from build123d import *

# Parameters (mm, degrees)
F0_W     = 800
F0_H     = 500
F1_DEPTH = 300
F2_T     = -1
F4_DEPTH = 798


with BuildPart() as f1:
    # F0 (on Top) → F1 (new body)
    with BuildSketch(Plane.XY):
        with Locations((400, 250)):
            Rectangle(F0_W, F0_H)
    extrude(amount=F1_DEPTH)

    # F2
    f2_openings = [f1.faces().sort_by_distance(p)[0] for p in [
        (400, 250, 300),
    ]]
    offset(amount=F2_T, openings=f2_openings)


with BuildPart() as f4:
    # F3 (on Right) → F4 (new body)
    with BuildSketch(Plane.YZ):
        Polygon((-25, 0), (0, 0), (0, 2), (-23, 2), (-23, 25), (-25, 25), align=None)
    extrude(amount=F4_DEPTH)


solid = f1.part
Geometry: final body of the model. Coordinates: model frame, mm. A direction names the side the tool comes from. Give positions to 0.01 mm unless a question says otherwise; leave off trailing zeros. Write each loop counter-clockwise with the first axis right and the second up, starting at its lowest first coordinate (ties: lowest second). Pieces come first, ordered by that corner, then holes. Notation, with made-up numbers: M 63.5,-6 L 67.5,-6 A38 cw 67.5,33 Z; hole C 39,-10.75 d4. An arc over 180 degrees is marked long. Answer in a Markdown table with one row per item. Add a question column.
(1) Section B-B on x = 729. Return loops of the section in (y, z).
(2) Ray query, line 1 (X direction, y = 458.5, z = 132); line 2 (Y direction, x = 276.5, z = 158.5); line 3 (Z direction, x = 385, y = 137). Return the intervals inside material, ascending.
(3) Section C-C on y = 325.5. Return loops of the section in (x, z).
(4) Section A-A on z = 123.5. Return loops of the section in (x, y), and give its area (3 significant figures).
(5) Reachability of faces 4 (the flat face through (394, 500, 148)), 5 (the flat face through (394, 1, 148)) from +Z, -Z, +X, -X, +Y, -Y: full face, straight path, thin tool, end or side. Return the list, or none.
(6) First-contact query: pin 1 (1 mm diameter, centred on x = 540.5, z = 172.5, fed in from -Y). Flat tip, straight axial feed; report the tip coordinate or a pass-through.
(7) Mould query, pull axis Y, two halves, no side actions, for faces 1 (the flat face through (394, 0, 148)), 2 (the flat face through (394, 253, 1)), 3 (the flat face through (800, 247, 148)). Classes: +Y half, -Y half, draft (parallel to the pull), parting line (faces both ways), or undercut.
Result set:
| question | item | result |
|---|---|---|
| 1 | outline | M 0,0 L 500,0 L 500,300 L 499,300 L 499,1 L 1,1 L 1,300 L 0,300 Z |
| 2 | line 1 | x = 0 to 1, 799 to 800 |
| 2 | line 2 | y = 0 to 1, 499 to 500 |
| 2 | line 3 | z = 0 to 1 |
| 3 | outline | M 0,0 L 800,0 L 800,300 L 799,300 L 799,1 L 1,1 L 1,300 L 0,300 Z |
| 4 | outline | M 0,0 L 800,0 L 800,500 L 0,500 Z; hole M 1,1 L 799,1 L 799,499 L 1,499 Z |
| 4 | area | 2,600 mm^2 |
| 5 | face 4 | +Z, -Z, +X, -X, +Y |
| 5 | face 5 | +Z |
| 6 | pin 1 | stops at y = 0 |
| 7 | face 1 | -Y half |
| 7 | face 2 | undercut |
| 7 | face 3 | draft |
